Geometry: final body of the model. Coordinates: model frame, mm. Face numbers are marked on the shaded views. A direction names the side the tool comes from. Coordinates: 2 decimals unless noted, no trailing zeros. Loops run counter-clockwise (first coordinate to the right, second up) from the corner with the lowest first, then second, coordinate; pieces in that order, holes last. Notation, with made-up numbers: (24.5, 52) - (76.5, 52) arc R22 ccw to (76.5, 80) - close; hole circle Ø5 at (24.5, -7.75). An arc over 180 degrees is marked (long way). Put each result on its own line as item: value. Start each with the question number.
1) Draft query along X for the marked faces 1, 2 and 3. Return one class per face: +X half, -X half, draft (parallel to the pull), parting line (faces both ways), or undercut.
2) Reachability of the marked faces 4, 5 and 6 from +Z, -Z, +X, -X, +Y, -Y: full face, straight path, thin tool, end or side. Return the list, or none.
3) Section A-A on y = 27.8. Output: boundary loops of the cut face in (x, z), and give its area (3 significant figures).
4) Section C-C on z = 7. Output: boundary loops of the cut face in (x, y).
5) Contact query for flat-ended pins moving along their axis: pin 1 Ø7 at (y, z) = (20.5, 8.5) entering from +X; pin 2 Ø3 at (x, z) = (23, 7) entering from -Y; pin 3 Ø7.5 at (x, z) = (4, 7.5) entering from +Y. Output: stop coordinate, or through.
6) Section B-B on x = 37. Output: boundary loops of the cut face in (y, z), and give its area (3 significant figures).
7) Material intervals for line 1 along X through (y, z) = (22, 7.75); line 2 along X through (y, z) = (18, 2); line 3 along Y through (x, z) = (16, 7), sorted ascending. Write a range as from..to.
8) Section D-D on y = 17.8. Output: boundary loops of the cut face in (x, z), and give its area (3 significant figures).
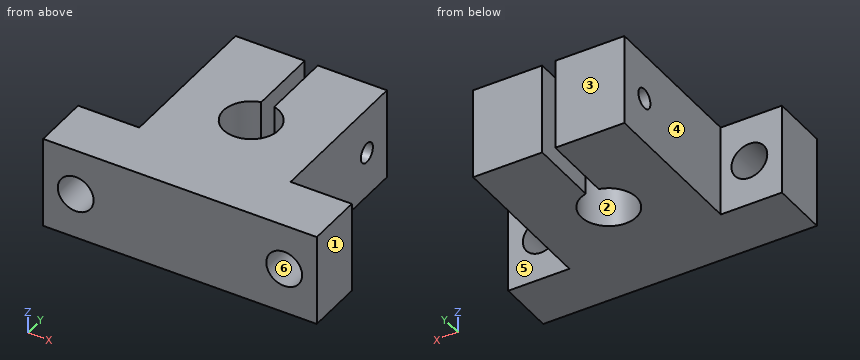
```python
from build123d import *

# Parameters (mm, degrees)
BOSS_EXTRUDE1_DEPTH = 14
SKETCH2_R           = 4.25
CUT_EXTRUDE1_DEPTH  = 56.098457329
SKETCH3_R           = 2.75
CUT_EXTRUDE2_DEPTH  = 51.388516183
SKETCH4_R           = 1.5
CUT_EXTRUDE3_DEPTH  = 49.323962746


with BuildPart() as part:
    # Sketch1 → Boss-Extrude1 (new body)
    with BuildSketch(Plane.XY):
        Polygon((0, 0), (42, 0), (42, 8.73752791), (32.609283578, 8.73752791), (32.609283578, 32.8), (22, 32.8), (22, 17.8), (20, 17.8), (20, 32.8), (9.390716422, 32.8), (9.390716422, 8.73752791), (0, 8.73752791), align=None)
    extrude(amount=BOSS_EXTRUDE1_DEPTH)

    # Sketch2 → Cut-Extrude1 (cut, through all)
    with BuildSketch(Plane.XY.offset(14)):
        with Locations((21, 17.8)):
            Circle(SKETCH2_R)
    extrude(amount=-CUT_EXTRUDE1_DEPTH, mode=Mode.SUBTRACT)

    # Sketch3 → Cut-Extrude2 (cut, through all)
    with BuildSketch(Plane(origin=(0, 8.73752791, 0), x_dir=(1, 0, 0), z_dir=(0, 1, 0))):
        with Locations(Location((5, -7, 0), (0, 0, 180))):
            Circle(SKETCH3_R)
        with Locations(Location((37, -7, 0), (0, 0, 180))):
            Circle(SKETCH3_R)
    extrude(amount=-CUT_EXTRUDE2_DEPTH, mode=Mode.SUBTRACT)

    # Sketch4 → Cut-Extrude3 (cut, through all)
    with BuildSketch(Plane(origin=(32.609283578, 0, 0), x_dir=(0, 0, -1), z_dir=(1, 0, 0))):
        with Locations((-7, 27.8)):
            Circle(SKETCH4_R)
    extrude(amount=-CUT_EXTRUDE3_DEPTH, mode=Mode.SUBTRACT)


solid = part.part
```
Answer block:
1. face 1: +X half
1. face 2: undercut
1. face 3: draft
2. face 4: +Z, -Z, -X, +Y
2. face 5: +Z, -Z, +X, +Y
2. face 6: +Y, -Y
3. outline: (9.39, 0) - (20, 0) - (20, 5.5) - (9.39, 5.5) - close; (9.39, 8.5) - (20, 8.5) - (20, 14) - (9.39, 14) - close; (22, 0) - (32.61, 0) - (32.61, 5.5) - (22, 5.5) - close; (22, 8.5) - (32.61, 8.5) - (32.61, 14) - (22, 14) - close
3. area: 233 mm²
4. outline: (0, 0) - (2.25, 0) - (2.25, 8.74) - (0, 8.74) - close; (7.75, 0) - (34.25, 0) - (34.25, 8.74) - (32.61, 8.74) - (32.61, 26.3) - (22, 26.3) - (22, 21.93) arc R4.25 cw (long way) to (20, 21.93) - (20, 26.3) - (9.39, 26.3) - (9.39, 8.74) - (7.75, 8.74) - close; (9.39, 29.3) - (20, 29.3) - (20, 32.8) - (9.39, 32.8) - close; (22, 29.3) - (32.61, 29.3) - (32.61, 32.8) - (22, 32.8) - close; (39.75, 0) - (42, 0) - (42, 8.74) - (39.75, 8.74) - close
5. pin 1: stops at x = 32.61
5. pin 2: stops at y = 0
5. pin 3: stops at y = 8.74
6. outline: (0, 0) - (8.74, 0) - (8.74, 4.25) - (0, 4.25) - close; (0, 9.75) - (8.74, 9.75) - (8.74, 14) - (0, 14) - close
6. area: 74.3 mm²
7. line 1: x = 9.39..20, 22..32.61
7. line 2: x = 9.39..16.75, 25.25..32.61
7. line 3: y = 0..26.3, 29.3..32.8
8. outline: (9.39, 0) - (16.75, 0) - (16.75, 14) - (9.39, 14) - close; (25.25, 0) - (32.61, 0) - (32.61, 14) - (25.25, 14) - close
8. area: 206 mm²
